The listing builds one solid part. Answer for the finished solid, in the listing's coordinates (mm). A direction names the side the tool comes from. Round coordinates to 2 decimals unless told otherwise and drop trailing zeros. Order: outer loops, then holes, each group sorted by start corner. A loop starts at its lowest first (then second) coordinate and runs counter-clockwise, first axis right, second up. Notation, with made-up numbers: (28.25, 2) -> (43.25, 2) arc R24 cw to (43.25, 26) -> close; hole circle Ø8 at (-30, 63.25). An arc over 180 degrees is marked (long way). Return JSON: item names as keys, results as strings. Group by question number.
(1) The part is cut by section A-A (z = 19.5). Determine the outline of the cut face in (x, y).
(2) Which of the six approach directions +Z, -Z, +X, -X, +Y, -Y give full straight-line access (tool end or side, diameter ignored) to faces 1 (the face through (-20.25, 0.5, 12.3)), 2 (the face through (-18.75, 0.5, 12.3)), 3 (the face through (-28.734, -11.808, 24.715))?
(3) Each of these flat-tipped pins is pushed along its axis until it touches: pin 1 (5 mm diameter, centred on x = -30.5, z = 11.5, fed in from +Y); pin 2 (0.9 mm diameter, centred on x = -18.5, z = 14.5, fed in from +Y); pin 3 (10 mm diameter, centred on y = -5, z = 17, fed in from -X). Where does it stop, or does it pass through?
(4) Consider line 1 (Y direction, x = -27.75, z = 19.75); line 2 (X direction, y = -6.5, z = 6.5); line 3 (X direction, y = -5.5, z = 9). Determine where each line is inside the solid, lowest interval first. Write a range as [from, to].
from build123d import *

# Parameters (mm, degrees)
F2_DEPTH = 25
F3_DEPTH = 25
F5_R     = 1


with BuildPart() as f2:
    # F0 (on Top) → F2 (new body)
    with BuildSketch(Plane.XY):
        Polygon((-17, 0), (-22, 0), (-37, -25), (-27, -25), align=None)
    extrude(amount=F2_DEPTH)

    # F1 (on Top) → F3 (join)
    with BuildSketch(Plane.XY):
        with BuildLine():
            Line((-20.25, 1), (-20.25, 0))
            Line((-20.25, 0), (-18.75, 0))
            Line((-18.75, 0), (-18.75, 1))
            ThreePointArc((-18.75, 1), (-19.5, 0.25), (-20.25, 1))
        make_face()
        with BuildLine():
            ThreePointArc((-18.75, 1), (-19.5, 1.75), (-20.25, 1))
            Line((-20.25, 1), (-18.75, 1))
        make_face()
        with BuildLine():
            Line((-18.75, 1), (-20.25, 1))
            ThreePointArc((-20.25, 1), (-19.5, 0.25), (-18.75, 1))
        make_face()
    extrude(amount=F3_DEPTH)

    # F5
    f5_edges = [f2.edges().sort_by_distance(p)[0] for p in [
        (-22, -12.5, 0),
        (-29.5, -12.5, 0),
        (-29.5, -12.5, 25),
        (-22, -12.5, 25),
        (-32, -25, 0),
        (-27, -25, 12.5),
        (-37, -25, 12.5),
        (-32, -25, 25),
    ]]
    fillet(f5_edges, radius=F5_R)


with BuildPart() as f2b:
    # F0 (on Top) → F2, piece 2 (new body)
    with BuildSketch(Plane.XY):
        Polygon((37, -25), (22, 0), (17, 0), (27, -25), align=None)
    extrude(amount=F2_DEPTH)

    # F1 (on Top) → F3, piece 2 (join)
    with BuildSketch(Plane.XY):
        with BuildLine():
            ThreePointArc((18.75, 1), (19.5, 0.25), (20.25, 1))
            ThreePointArc((20.25, 1), (19.5, 1.75), (18.75, 1))
        make_face()
        with BuildLine():
            Line((20.25, 0), (20.25, 1))
            ThreePointArc((20.25, 1), (19.5, 0.25), (18.75, 1))
            Line((18.75, 1), (18.75, 0))
            Line((18.75, 0), (20.25, 0))
        make_face()
    extrude(amount=F3_DEPTH)


solid = f2.part
Answer below:
{
 "1": {"outline": "(-36.09, -23.49) arc R1 ccw to (-35.23, -25) -> (-27.68, -25) arc R1 ccw to (-26.75, -24.37) -> (-17, 0) -> (-18.75, 0) -> (-18.75, 1) arc R0.75 ccw to (-20.25, 1) -> (-20.25, 0) -> (-22, 0) -> close"},
 "2": {"face 1": "+Z, -Z, -X, +Y", "face 2": "+Z, -Z, +X, +Y", "face 3": "+Z, -X, +Y"},
 "3": {"pin 1": "stops at y = -10", "pin 2": "stops at y = 1.51", "pin 3": "stops at x = -28"},
 "4": {"line 1": "y = [-25, -9.58]", "line 2": "x = [-25.9, -19.6]", "line 3": "x = [-25.3, -19.2]"}
}
